The listing builds one solid part. Answer for the finished solid, in the listing's coordinates (mm). Face numbers are marked on the shaded views. Give positions to 0.01 mm unless a question says otherwise; leave off trailing zeros. Loops run counter-clockwise (first coordinate to the right, second up) from the corner with the lowest first, then second, coordinate; pieces in that order, holes last.
Item 1: Consider line 1 along Z through (x, y) = (9.55, 0); line 2 along Z through (x, y) = (2.75, 0). Determine where each line is inside the solid, lowest interval first.
Item 2: Section D-D, the plane x = 11.75 is taken. Give the vertices of the cut face in (y, z).
Item 3: Section C-C, the plane x = 2.75 is taken. Give the vertices of the cut face in (y, z).
Item 4: Each of these flat-tipped pins is pushed along its axis until it touches: pin 1 Ø1.8 at (y, z) = (1, 0) entering from -X; pin 2 Ø1 at (x, y) = (9, -3.5) entering from -Z; pin 3 Ø2 at (x, z) = (5, 16) entering from -Y. Where does it stop, or does it pass through?
Item 5: The mould has two halves that part along Z. Classify the marked faces 1, 2, 3 and 4: pulls with the +Z half, pulls with the -Z half, needs draft (parallel to the pull), parting line crosses it, or undercut.
Item 6: Section A-A, the plane z = 0 is taken. Give the vertices of the cut face in (x, y) (3 decimals).
from build123d import *

# Parameters (mm, degrees)
F2_R     = 3
F3_DEPTH = 0.889


with BuildPart() as f1:
    # F0 (on Front) → F1 (revolve)
    with BuildSketch(Plane.XZ):
        with BuildLine():
            Line((0, 20.955), (0, 19.05))
            Line((0, 19.05), (8.89, 19.05))
            Line((8.89, 19.05), (8.89, 0))
            Line((8.89, 0), (12.7, 0))
            Line((12.7, 0), (12.7, 20.955))
            ThreePointArc((12.7, 20.955), (12.142038, 22.302038), (10.795, 22.86))
            Line((10.795, 22.86), (1.905, 22.86))
            ThreePointArc((1.905, 22.86), (0.557962, 22.302038), (0, 20.955))
        make_face()
    revolve(axis=Axis((2.430882, 0, 0), (1, 0, 0)))

    # F2 (on face) → F3 (cut)
    with BuildSketch(Plane(origin=(8.89, 0, 0), x_dir=(0, -1, 0), z_dir=(-1, 0, 0))):
        Circle(F2_R)
    extrude(amount=-F3_DEPTH, mode=Mode.SUBTRACT)


solid = f1.part
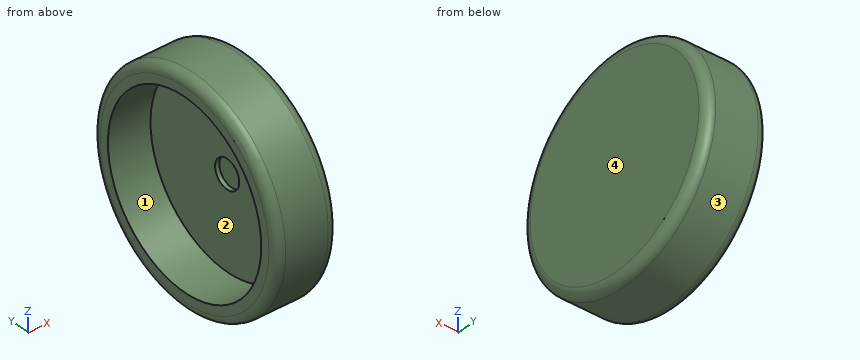
Worked answers:
1. line 1: z = -22.86 to -3, 3 to 22.86
1. line 2: z = -22.86 to -19.05, 19.05 to 22.86
2. outline: circle Ø45.21 at (0, 0)
3. outline: circle Ø45.72 at (0, 0); hole circle Ø38.1 at (0, 0)
4. pin 1: stops at x = 9.78
4. pin 2: stops at z = -22.66
4. pin 3: stops at y = -17.25
5. face 1: undercut
5. face 2: undercut
5. face 3: parting line crosses it
5. face 4: needs draft
6. outline: (0, -20.955) arc R1.905 ccw to (1.905, -22.86) - (10.795, -22.86) arc R1.905 ccw to (12.7, -20.955) - (12.7, 20.955) arc R1.905 ccw to (10.795, 22.86) - (1.905, 22.86) arc R1.905 ccw to (0, 20.955) - (0, 19.05) - (8.89, 19.05) - (8.89, 3) - (9.779, 3) - (9.779, -3) - (8.89, -3) - (8.89, -19.05) - (0, -19.05) - close
